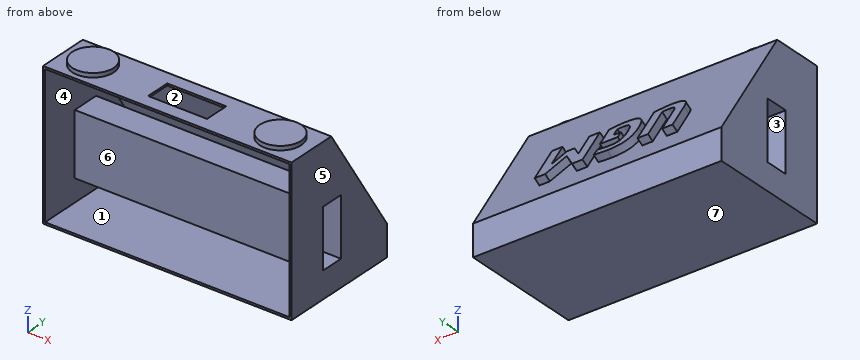
```python
from build123d import *

# Parameters (mm, degrees)
SKETCH2_W           = 28.306958552
SKETCH2_H           = 11.453917389
BOSS_EXTRUDE1_DEPTH = 120
SHELL1_T            = -1
SKETCH3_R           = 10
BOSS_EXTRUDE3_DEPTH = 2
BOSS_EXTRUDE4_DEPTH = 3.5
SKETCH5_W           = 28.5
SKETCH5_H           = 12
CUT_EXTRUDE1_DEPTH  = 3.5


with BuildPart() as part:
    # Sketch2 → Boss-Extrude1 (new body)
    with BuildSketch(Plane(origin=(0, 0, 0), x_dir=(0, 0, -1), z_dir=(1, 0, 0))):
        Polygon((0, 0), (-70, 0), (-70, 25), (-15, 60), (0, 60), align=None)
        with Locations((-27.013142097, 25.361400481)):
            Rectangle(SKETCH2_W, SKETCH2_H, mode=Mode.SUBTRACT)
    extrude(amount=BOSS_EXTRUDE1_DEPTH)

    # Shell1
    shell1_openings = [part.faces().sort_by_distance(p)[0] for p in [
        (60, 0, 35),
    ]]
    offset(amount=SHELL1_T, openings=shell1_openings, kind=Kind.INTERSECTION)

    # Sketch3 → Boss-Extrude3 (add)
    with BuildSketch(Plane.XY.offset(70)):
        with Locations(Location((14.460503184, 12.622362689, 0), (0, 0, 180))):
            Circle(SKETCH3_R)
        with Locations(Location((104.984833399, 12.622362689, 0), (0, 0, 180))):
            Circle(SKETCH3_R)
    extrude(amount=BOSS_EXTRUDE3_DEPTH)

    # Sketch4 → Boss-Extrude4 (add)
    with BuildSketch(Plane(origin=(0, 49.5, 31.5), x_dir=(1, 0, 0), z_dir=(0, 0.8436614877321076, 0.5368754921931594))):
        with BuildLine():
            Line((31.495555556, 7.28159519), (31.495555556, -6.582571477))
            add(Edge.make_bspline(
                [(31.495555556, -6.582571477), (31.497647327, -6.716452984), (31.501705357, -6.976182729), (31.545429981, -7.349903275), (31.620254564, -7.694330516), (31.725797404, -8.007755097), (31.85843149, -8.292023496), (32.017035255, -8.549104595), (32.213580402, -8.769410834), (32.514616663, -9.027825691), (32.965416445, -9.28279655), (33.584183504, -9.496713073), (34.290093212, -9.63052642), (34.790447792, -9.644416316), (35.054201389, -9.651738144)],
                knots=[0, 0, 0, 0, 0.892406739, 1.731266554, 2.504144536, 3.238722317, 3.931504629, 4.59227798, 5.245079782, 5.891448425, 7.23122422, 8.666543773, 10.242823978, 12, 12, 12, 12], degree=3))
            add(Edge.make_bspline(
                [(35.054201389, -9.651738144), (35.371915661, -9.647351405), (35.987813895, -9.638847586), (36.738630256, -9.567280303), (37.293698587, -9.49725925), (37.65928604, -9.438298039), (37.980921199, -9.384777988), (38.177949016, -9.338130022), (38.268888889, -9.316599255)],
                knots=[0, 0, 0, 0, 1.765444015, 3.422363889, 4.188491736, 4.874885831, 5.480693936, 6, 6, 6, 6], degree=3))
            Line((38.268888889, -9.316599255), (38.268888889, 7.28159519))
            Line((38.268888889, 7.28159519), (43.348888889, 7.28159519))
            Line((43.348888889, 7.28159519), (43.348888889, -12.04621731))
            add(Edge.make_bspline(
                [(43.348888889, -12.04621731), (43.096189549, -12.108469187), (42.560643091, -12.240399773), (41.708016667, -12.438755514), (40.760798722, -12.647829999), (39.72837029, -12.878596561), (38.613480039, -13.080203608), (37.426291642, -13.215675326), (36.175767269, -13.309081819), (35.320438728, -13.316715841), (34.882222222, -13.320627033)],
                knots=[0, 0, 0, 0, 0.727273077, 1.541311979, 2.446196716, 3.437977513, 4.497566055, 5.610312566, 6.77567458, 8, 8, 8, 8], degree=3))
            add(Edge.make_bspline(
                [(34.882222222, -13.320627033), (34.504262876, -13.314914498), (33.778113064, -13.30393936), (32.735267925, -13.21513127), (31.783524991, -13.074414795), (30.921420697, -12.867783559), (30.146372308, -12.601500494), (29.446115226, -12.292080995), (28.830068546, -11.917580353), (28.282939924, -11.498254497), (27.818160366, -11.016573216), (27.419646968, -10.485522985), (27.09211977, -9.899752382), (26.836782361, -9.259995921), (26.649530032, -8.569422805), (26.515550652, -7.834688866), (26.428130138, -7.052093695), (26.41983098, -6.515200865), (26.415555556, -6.238613144)],
                knots=[0, 0, 0, 0, 1.424825587, 2.737428892, 3.942915469, 5.049168469, 6.074440888, 7.029373324, 7.929451529, 8.786387261, 9.62117339, 10.444717279, 11.283376038, 12.14372783, 13.035182641, 13.976509509, 14.957571058, 16, 16, 16, 16], degree=3))
            Line((26.415555556, -6.238613144), (26.415555556, 7.28159519))
            Line((26.415555556, 7.28159519), (31.495555556, 7.28159519))
        make_face()
        with BuildLine():
            add(Edge.make_bspline(
                [(64.356805556, 3.224650745), (64.152697046, 3.265479221), (63.723461512, 3.351340574), (63.041961215, 3.462909191), (62.29583847, 3.579450279), (61.212104745, 3.717973311), (59.811209671, 3.867682682), (58.676089338, 3.885843376), (58.108229167, 3.894928523)],
                knots=[0, 0, 0, 0, 0.595250767, 1.251798765, 1.974755809, 2.75480843, 4.376546534, 6, 6, 6, 6], degree=3))
            add(Edge.make_bspline(
                [(58.108229167, 3.894928523), (57.866952661, 3.891547515), (57.40238535, 3.885037532), (56.73040283, 3.811402786), (56.110259397, 3.700425968), (55.539401639, 3.541723685), (55.018275771, 3.335491675), (54.545861683, 3.07246126), (54.119187516, 2.758203357), (53.73932494, 2.388321122), (53.411594136, 1.958862272), (53.126376495, 1.47215962), (52.890281289, 0.923783122), (52.700878804, 0.312954851), (52.558002514, -0.361956903), (52.452465427, -1.105813902), (52.392758083, -1.921988909), (52.384365104, -2.490252469), (52.38, -2.785800644)],
                knots=[0, 0, 0, 0, 1.133437581, 2.182384265, 3.172832728, 4.091362303, 4.962372543, 5.800406583, 6.625239699, 7.445925786, 8.283247732, 9.156419393, 10.090711351, 11.082628234, 12.157104624, 13.32943025, 14.61106347, 16, 16, 16, 16], degree=3))
            add(Edge.make_bspline(
                [(52.38, -2.785800644), (52.384196723, -3.118101326), (52.392226664, -3.753919963), (52.453172237, -4.660728623), (52.551999251, -5.475433806), (52.690933664, -6.199839009), (52.872671982, -6.841126791), (53.08689051, -7.407019826), (53.332449966, -7.901073543), (53.612537323, -8.323257374), (53.928446967, -8.677755377), (54.282503677, -8.965737434), (54.662550063, -9.204286947), (55.080076889, -9.375736284), (55.526049387, -9.495182682), (55.994151932, -9.589102), (56.490115847, -9.642084068), (56.827818042, -9.648460705), (57.001388889, -9.651738144)],
                knots=[0, 0, 0, 0, 1.673454126, 3.201959486, 4.57468475, 5.80438305, 6.912760951, 7.927383973, 8.847752408, 9.685453157, 10.471760189, 11.229097717, 11.976932424, 12.723483608, 13.492240552, 14.299457069, 15.125961629, 16, 16, 16, 16], degree=3))
            add(Edge.make_bspline(
                [(57.001388889, -9.651738144), (57.242566033, -9.648444955), (57.747594043, -9.641548975), (58.513397038, -9.57931793), (59.271728701, -9.503258107), (59.766374362, -9.442370781), (60, -9.413613144)],
                knots=[0, 0, 0, 0, 0.961374604, 2.013130658, 3.061583563, 4, 4, 4, 4], degree=3))
            Line((60, -9.413613144), (60, -5.136182588))
            Line((60, -5.136182588), (56.494270833, -5.136182588))
            Line((56.494270833, -5.136182588), (56.494270833, -1.467293699))
            Line((56.494270833, -1.467293699), (65.08, -1.467293699))
            Line((65.08, -1.467293699), (65.08, -12.121182588))
            add(Edge.make_bspline(
                [(65.08, -12.121182588), (64.839162189, -12.185262296), (64.319249791, -12.32359537), (63.48922284, -12.523718247), (62.569821699, -12.718386963), (61.587737426, -12.910998872), (60.550412746, -13.071297466), (59.476477777, -13.210276189), (58.380235988, -13.301780667), (57.645379742, -13.314359172), (57.279201389, -13.320627033)],
                knots=[0, 0, 0, 0, 0.755794281, 1.631582744, 2.588976596, 3.605760095, 4.666252689, 5.771549146, 6.889564499, 8, 8, 8, 8], degree=3))
            add(Edge.make_bspline(
                [(57.279201389, -13.320627033), (56.889513874, -13.314630804), (56.129685347, -13.302939114), (55.022260593, -13.214317278), (53.977001934, -13.068115209), (52.991445011, -12.873539155), (52.074025504, -12.591714386), (51.225843147, -12.226132778), (50.455091299, -11.762640122), (49.866957383, -11.308619162), (49.437870421, -10.898615459), (49.137720463, -10.560848798), (48.853553039, -10.197957504), (48.591133595, -9.806679294), (48.346191057, -9.388659543), (48.123831144, -8.944055848), (47.914563451, -8.473869404), (47.724821117, -7.97527371), (47.556866599, -7.443814271), (47.413113475, -6.879657909), (47.287128379, -6.28138145), (47.19474622, -5.647516108), (47.11363965, -4.980235153), (47.05618482, -4.280100825), (47.027329608, -3.5445168), (47.021016482, -3.043055789), (47.017777778, -2.785800644)],
                knots=[0, 0, 0, 0, 1.640766254, 3.199232612, 4.674144897, 6.083442838, 7.424489995, 8.707789567, 9.962455245, 11.201775806, 11.827763747, 12.458962377, 13.10278022, 13.767126437, 14.441204247, 15.14151096, 15.859189204, 16.60751955, 17.386599082, 18.204749424, 19.058103002, 19.959719952, 20.900938005, 21.888338343, 22.916693792, 24, 24, 24, 24], degree=3))
            add(Edge.make_bspline(
                [(47.017777778, -2.785800644), (47.020628796, -2.546168569), (47.026211518, -2.076932884), (47.06082015, -1.386885284), (47.122591725, -0.727947698), (47.206582105, -0.098344535), (47.311213943, 0.502492016), (47.441555443, 1.074288834), (47.602601185, 1.6150534), (47.838760081, 2.288312532), (48.193444972, 3.068600834), (48.700360125, 3.924608099), (49.295402807, 4.679017259), (49.968787038, 5.339138985), (50.718272671, 5.907422518), (51.547607876, 6.379904626), (52.447590869, 6.770661477), (53.42293726, 7.065844151), (54.461089467, 7.286413605), (55.555206299, 7.449289699), (56.707046728, 7.548152282), (57.49360801, 7.55851077), (57.8965625, 7.563817412)],
                knots=[0, 0, 0, 0, 0.830523012, 1.626289114, 2.393765786, 3.123613252, 3.827153004, 4.506826794, 5.154833919, 5.781607132, 6.978567384, 8.118716626, 9.221456624, 10.298587739, 11.378606288, 12.471761326, 13.598907335, 14.771984998, 15.997030156, 17.274417513, 18.603687055, 20, 20, 20, 20], degree=3))
            add(Edge.make_bspline(
                [(57.8965625, 7.563817412), (58.181795123, 7.561761396), (58.776171037, 7.557477012), (59.687545429, 7.503809961), (60.625305238, 7.434475444), (61.555873436, 7.350783248), (62.453370731, 7.257685343), (63.289275957, 7.142331595), (64.031358868, 7.030292802), (64.486422582, 6.939124145), (64.691944444, 6.897949356)],
                knots=[0, 0, 0, 0, 1.001170159, 2.086267066, 3.203892355, 4.302208362, 5.366093373, 6.37097994, 7.264280522, 8, 8, 8, 8], degree=3))
            Line((64.691944444, 6.897949356), (64.356805556, 3.224650745))
        make_face()
        Polygon((79.574756944, -6.913300644), (74.957777778, -0.113508977), (74.957777778, -13.03840481), (69.877777778, -13.03840481), (69.877777778, 7.28159519), (74.957777778, 7.28159519), (81.462118056, -2.252224255), (87.94, 7.28159519), (93.02, 7.28159519), (93.02, -13.03840481), (87.94, -13.03840481), (87.94, -0.113508977), (83.323020833, -6.913300644), align=None)
    extrude(amount=BOSS_EXTRUDE4_DEPTH)

    # Sketch5 → Cut-Extrude1 (cut)
    with BuildSketch(Plane.XY.offset(70)):
        with Locations((60, 12.5)):
            Rectangle(SKETCH5_W, SKETCH5_H)
    extrude(amount=-CUT_EXTRUDE1_DEPTH, mode=Mode.SUBTRACT)


solid = part.part
```
The listing builds one solid part. Answer for the finished solid, in the listing's coordinates (mm). Face numbers are marked on the shaded views. A direction names the side the tool comes from. Coordinates: 2 decimals unless noted, no trailing zeros. Order: outer loops, then holes, each group sorted by start corner. A loop starts at its lowest first (then second) coordinate and runs counter-clockwise, first axis right, second up. Notation, with made-up numbers: M 3,17 L 54,17 A25 ccw 54,34 Z; hole C -3.5,-7 d2. An arc over 180 degrees is marked long. Answer as a JSON object with one key per item and string values. Group by question number.
1. A tool of negligible diameter and unlimited length cuts with its end or side. For the marked faces 1, 2 and 3, from which of +Z, -Z, +X, -X, +Y, -Y can it reach the whole face along a straight path? Write none if from no direction.
2. Section B-B on y = 35 is taken. Write down the section's boundary in (x, z).
3. Straight lines are drawn through the part: line 1 (Z direction, x = 31, y = 20); line 2 (X direction, y = 6.5, z = 12); line 3 (Z direction, x = 80, y = 11). For each, find the intervals that lie inside material, in ascending order.
4. Section A-A on x = 104 is taken. Write down the section's boundary in (y, z), then the cut area to 3 significant figures.
5. Flat-ended cylindrical pins translate along their axes: P1, Ø10, axis at y = 23.5, z = 63, coming from the -X side; P2, Ø1.5, axis at x = 52, z = 42, coming from the +Y side; P3, Ø0.5, axis at x = 65, z = 69.5, coming from the +Y side; P4, Ø12.5, axis at x = 40.5, y = 13.5, coming from the +Z side. Find the tip coordinate at first contact, or state that the pin passes through.
6. Determine the mould class of the marked faces 4, 5, 6 and 7 for opening direction X: released by +X, released by -X, zero draft, split by the parting line, or undercut.
7. Section C-C on z = 9.5 is taken. Write down the section's boundary in (x, y).
8. Section D-D on x = 28 is taken. State how many separate pieces and enclosed holes the cut face has, then the cut area to 3 significant figures.
Values follow:
{
 "1": {"face 1": "-Y", "face 2": "none", "face 3": "+X, -X"},
 "2": {"outline": "M 0,0 L 120,0 L 120,54.29 L 0,54.29 Z; hole M 1,1 L 119,1 L 119,52.42 L 1,52.42 Z"},
 "3": {"line 1": "0 to 1, 11.86 to 12.86, 41.17 to 42.17, 69 to 70", "line 2": "0 to 1, 119 to 120", "line 3": "0 to 1, 69 to 70"},
 "4": {"outline": "M 0,0 L 60,0 L 60,15 L 25,70 L 22.57,70 L 22.57,72 L 2.67,72 L 2.67,70 L 0,70 L 0,69 L 24.45,69 L 59,14.71 L 59,1 L 0,1 Z; M 18.63,11.86 L 32.09,11.86 L 32.09,42.17 L 18.63,42.17 Z; hole M 19.63,12.86 L 31.09,12.86 L 31.09,41.17 L 19.63,41.17 Z", "area": "287 mm2"},
 "5": {"P1": "x = 0", "P2": "y = 47.44", "P3": "y = 25.48", "P4": "z = 70"},
 "6": {"face 4": "undercut", "face 5": "released by +X", "face 6": "undercut", "face 7": "zero draft"},
 "7": {"outline": "M 0,0 L 1,0 L 1,59 L 119,59 L 119,0 L 120,0 L 120,60 L 0,60 Z"},
 "8": {"separate pieces": "2", "enclosed holes": "1", "area": "312 mm2"}
}
